```python
from build123d import *

# Parameters (mm, degrees)
SKETCH1_W           = 310.63946
SKETCH1_H           = 92.869200088
BOSS_EXTRUDE1_DEPTH = 143.6878
SKETCH2_R           = 6.35
CUT_EXTRUDE1_DEPTH  = 355.637485755
SKETCH3_W           = 310.82742
SKETCH3_H           = 12.7
CUT_EXTRUDE2_DEPTH  = 25.4


with BuildPart() as part:
    # Sketch1 → Boss-Extrude1 (new body)
    with BuildSketch(Plane(origin=(0, 0, 0), x_dir=(1, 0, 0), z_dir=(0, 1, 0))):
        with Locations((155.31973, 46.434600044)):
            Rectangle(SKETCH1_W, SKETCH1_H)
    extrude(amount=BOSS_EXTRUDE1_DEPTH)

    # Sketch2 → Cut-Extrude1 (cut, through all)
    with BuildSketch(Plane(origin=(0, 143.6878, 0), x_dir=(1, 0, 0), z_dir=(0, 1, 0))):
        with Locations(Location((46.7106, 45.72, 0), (0, 0, 270))):
            Circle(SKETCH2_R)
        with Locations(Location((263.92886, 45.72, 0), (0, 0, 90))):
            Circle(SKETCH2_R)
    extrude(amount=-CUT_EXTRUDE1_DEPTH, mode=Mode.SUBTRACT)

    # Sketch3 → Cut-Extrude2 (cut)
    with BuildSketch(Plane(origin=(0, 143.6878, 0), x_dir=(1, 0, 0), z_dir=(0, 1, 0))):
        with Locations((155.41371, 87.68842)):
            Rectangle(SKETCH3_W, SKETCH3_H)
    cut_extrude2 = extrude(amount=-CUT_EXTRUDE2_DEPTH, mode=Mode.SUBTRACT)

    # Mirror1: Cut-Extrude2 across plane
    add(cut_extrude2.mirror(Plane.ZX.offset(71.8439)), mode=Mode.SUBTRACT)


solid = part.part
```
For this review, take the finished solid that the model builds, in its own axes (mm). A direction names the side the tool comes from. Coordinates: 2 decimals unless noted, no trailing zeros. Loops run counter-clockwise (first coordinate to the right, second up) from the corner with the lowest first, then second, coordinate; pieces in that order, holes last. Notation, with made-up numbers: (-28, -30.5) -> (31, -30.5) arc R38 ccw to (31, 7.5) -> close; hole circle Ø5 at (-8.75, -34). An arc over 180 degrees is marked (long way). Return JSON: item names as keys, results as strings. Group by question number.
(1) Consider section C-C, the plane y = 134.5. Give the boundary of the cut face in (x, z).
(2) Tool access review of faces 5 (the flat face through (310.639, 71, -46)), 6 (the flat face through (153, 131, -81.338)), 7 (the flat face through (153, 25.4, -87)): name each direction out of +Z, -Z, +X, -X, +Y, -Y from which nothing blocks a thin tool from reaching the whole face with its end or side.
(3) For pin 1 Ø12.5 at (x, z) = (118, -87) entering from -Y; pin 2 Ø9 at (x, z) = (171.5, -89) entering from +Y; pin 3 Ø1 at (x, y) = (212, 124.5) entering from -Z; pin 4 Ø11.5 at (x, z) = (263.93, -45.72) entering from -Y, all flat-tipped, find the tip position at first contact; note any pin that passes through.
(4) To check wall thickness, follow L1, parallel to X at y = 67.5, z = -45.72; L2, parallel to X at y = 41, z = -46.5; L3, parallel to Y at x = 31.5, z = -87.5. State the ranges of each line that lie inside material, in increasing order.
(5) Consider section B-B, the plane x = 248.5. Give the boundary of the cut face in (y, z), plus the area to 3 significant figures.
(6) Mouldability with a two-part tool opening along Z and no side actions: class faces 1 (the flat face through (153, 118.288, -87)), 2 (the cylindrical face through (53.007, 72.85, -46.547)), 3 (the flat face through (153, 71, 0)), 4 (the cylindrical face through (257.633, 72.85, -44.893)) as pulls with the +Z half, pulls with the -Z half, needs draft (parallel to the pull), parting line crosses it, or undercut.
(7) Consider section A-A, the plane z = -45.72. Give the boundary of the cut face in (x, y).
Results below:
{
 "1": {"outline": "(0, -81.34) -> (310.64, -81.34) -> (310.64, 0) -> (0, 0) -> close; hole circle Ø12.7 at (46.71, -45.72); hole circle Ø12.7 at (263.93, -45.72)"},
 "2": {"face 5": "+Z, -Z, +X, +Y, -Y", "face 6": "-Z, +X, -X, +Y", "face 7": "-Z, +X, -X, -Y"},
 "3": {"pin 1": "stops at y = 0", "pin 2": "stops at y = 118.29", "pin 3": "stops at z = -81.34", "pin 4": "passes through"},
 "4": {"L1": "x = 0 to 40.36, 53.06 to 257.58, 270.28 to 310.64", "L2": "x = 0 to 40.41, 53.01 to 257.63, 270.23 to 310.64", "L3": "y = 25.4 to 118.29"},
 "5": {"outline": "(0, -81.34) -> (25.4, -81.34) -> (25.4, -92.87) -> (118.29, -92.87) -> (118.29, -81.34) -> (143.69, -81.34) -> (143.69, 0) -> (0, 0) -> close", "area": "12,800 mm2"},
 "6": {"face 1": "needs draft", "face 2": "undercut", "face 3": "pulls with the +Z half", "face 4": "undercut"},
 "7": {"outline": "(0, 0) -> (40.36, 0) -> (40.36, 143.69) -> (0, 143.69) -> close; (53.06, 0) -> (257.58, 0) -> (257.58, 143.69) -> (53.06, 143.69) -> close; (270.28, 0) -> (310.64, 0) -> (310.64, 143.69) -> (270.28, 143.69) -> close"}
}
